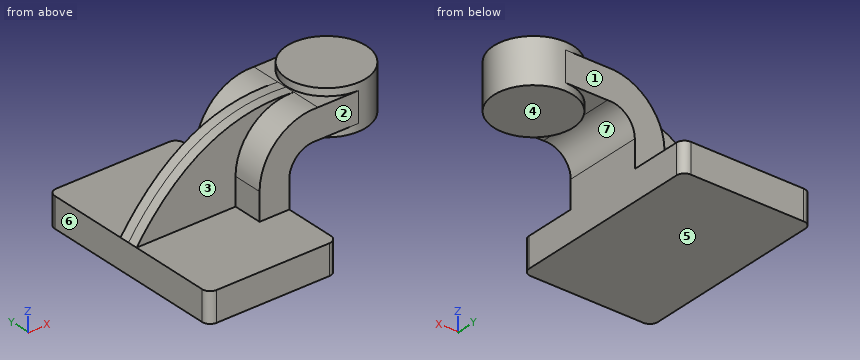
from build123d import *

# Parameters (mm, degrees)
F1_DEPTH = 63.5
F0_W     = 25.4
F0_H     = 19.05
F2_DEPTH = 25.4
F3_DEPTH = 6.35
F5_R     = 5.08


# Not quite as in the source:
# - a length typed as a fraction of an inch, garbled in the dataset ("3 / 203.2 mm" for 3/8 in), is restored


with BuildPart() as f1:
    # F0 (on Front) → F1 (new body, symmetric)
    with BuildSketch(Plane.XZ):
        Polygon((-41.275, -9.525), (41.275, -9.525), (41.275, 9.525), (22.225, 9.525), (-41.275, 9.525), align=None)
    extrude(amount=F1_DEPTH, both=True)

    # F0 (on Front) → F2 (join, symmetric)
    with BuildSketch(Plane.XZ):
        with BuildLine():
            Line((22.225, 9.525), (41.275, 9.525))
            Line((41.275, 9.525), (41.275, 27.1006073004))
            ThreePointArc((41.275, 27.1006073004), (46.5301853034, 38.9004022482), (58.8164375824, 42.8879))
            Line((58.8164375824, 42.8879), (60.325, 42.8879))
            Line((60.325, 42.8879), (60.325, 61.9379))
            Line((60.325, 61.9379), (59.6235930061, 61.9379))
            ThreePointArc((59.6235930061, 61.9379), (33.3449019193, 52.6558989318), (22.225, 27.1006073004))
            Line((22.225, 27.1006073004), (22.225, 9.525))
        make_face()
        with Locations((73.025, 52.4129)):
            Rectangle(F0_W, F0_H)
    extrude(amount=F2_DEPTH, both=True)

    # F0 (on Front) → F3 (join, symmetric)
    with BuildSketch(Plane.XZ):
        with BuildLine():
            add(Edge.make_bspline(
                [(59.6235930061, 61.9379), (21.0421923548, 65.1707053185), (-12.7928890288, 50.4826121032), (-41.275, 9.525)],
                knots=[0, 0, 0, 0, 113.6997720183, 113.6997720183, 113.6997720183, 113.6997720183], degree=3))
            Line((-41.275, 9.525), (22.225, 9.525))
            Line((22.225, 9.525), (22.225, 27.1006073004))
            ThreePointArc((22.225, 27.1006073004), (33.3449019193, 52.6558989318), (59.6235930061, 61.9379))
        make_face()
    extrude(amount=F3_DEPTH, both=True)

    # F0 (on Front) → F4 (revolve)
    with BuildSketch(Plane.XZ):
        Polygon((85.725, 66.675), (85.725, 61.9379), (85.725, 42.8879), (85.725, 38.1), (111.125, 38.1), (111.125, 66.675), align=None)
    revolve(axis=Axis((85.725, 0, 52.3875), (0, 0, -1)))

    # F5
    f5_edges = [f1.edges().sort_by_distance(p)[0] for p in [
        (41.275, -63.5, 0),
        (-41.275, -63.5, 0),
        (41.275, 63.5, 0),
        (-41.275, 63.5, 0),
    ]]
    fillet(f5_edges, radius=F5_R)


solid = f1.part
CAD build for the part. Positions are in the model's coordinates, mm. Face numbers are marked on the shaded views. A direction names the side the tool comes from. Give positions to 0.01 mm unless a question says otherwise; leave off trailing zeros. Loops run counter-clockwise (first coordinate to the right, second up) from the corner with the lowest first, then second, coordinate; pieces in that order, holes last. Notation, with made-up numbers: M -12,49.25 L 25,49.25 A23 ccw 25,86.25 Z; hole C -18,20.5 d5. An arc over 180 degrees is marked long. Write each question's results on one line, items separated by ' | '.
Q1. Band-saw the part on A-A on y = -15. Write the cut outline in (x, z) (3 decimals), and give its area (3 significant figures).
Geometry check:
outline: M -41.275,-9.525 L 41.275,-9.525 L 41.275,27.101 A15.875 cw 58.816,42.888 L 65.227,42.888 L 65.227,38.1 L 106.223,38.1 L 106.223,66.675 L 65.227,66.675 L 65.227,61.938 L 59.624,61.938 A34.925 ccw 22.225,27.101 L 22.225,9.525 L -41.275,9.525 Z | area: 3,990 mm²
Q2. Band-saw the part on B-B on y = 19. Write the cut outline in (x, z) (3 decimals).
Geometry check:
outline: M -41.275,-9.525 L 41.275,-9.525 L 41.275,27.101 A15.875 cw 58.816,42.888 L 68.868,42.888 L 68.868,38.1 L 102.582,38.1 L 102.582,66.675 L 68.868,66.675 L 68.868,61.938 L 59.624,61.938 A34.925 ccw 22.225,27.101 L 22.225,9.525 L -41.275,9.525 Z
Q3. Probe probe 1 along Y at (x, z) = (-31.5, 11.5); probe 2 along Z at (x, y) = (-20, 34) (3 decimals); probe 3 along X at (y, z) = (10.5, 20) (3 decimals). List the from-to ranges inside material, lowest first.
Geometry check:
probe 1: y = -6.35 to 6.35 | probe 2: z = -9.525 to 9.525 | probe 3: x = 22.225 to 41.275
Q4. Band-saw the part on C-C on y = 41.5. Write the cut outline in (x, z) (3 decimals).
Geometry check:
outline: M -41.275,-9.525 L 41.275,-9.525 L 41.275,9.525 L -41.275,9.525 Z
Q5. Which spindle directions (+Z, -Z, +X, -X, +Y, -Y) get a long thin tool onto all of the face, cutting with end or side? Do the marked faces 1, 2, 3 and 4. Say none if no direction does.
Geometry check:
face 1: +Z, +X, -X, +Y | face 2: +Z, +X, -X, -Y | face 3: +Z, -X, -Y | face 4: -Z, +X, +Y, -Y
Q6. Mould opens along X. For the marked faces 5, 6 and 7 say: pulls with the +X half, pulls with the -X half, needs draft (parallel to the pull), parting line crosses it, or undercut.
Geometry check:
face 5: needs draft | face 6: pulls with the -X half | face 7: undercut
Q7. Flat gauge pins, fed straight in: P1, Ø5, axis at x = 9, z = 38.5, coming from the -Y side; P2, Ø6, axis at y = 19, z = 41.5, coming from the -X side; P3, Ø5.5, axis at y = 18.5, z = 21, coming from the -X side (3 decimals). Where does each tip first touch, or does it go through?
Geometry check:
P1: stops at y = -6.35 | P2: stops at x = 24.14 | P3: stops at x = 22.225
